Geometry check sheet. Reference: the model listing, model coordinates, mm. A direction names the side the tool comes from. Coordinates: 2 decimals unless noted, no trailing zeros. Write each loop counter-clockwise with the first axis right and the second up, starting at its lowest first coordinate (ties: lowest second). Pieces come first, ordered by that corner, then holes. Notation, with made-up numbers: (12.5, 36) -> (31.5, 36) arc R13 cw to (31.5, 48) -> close; hole circle Ø1 at (73, -22). An arc over 180 degrees is marked (long way). One line per question, with ' | ' between items.
```python
from build123d import *

# Parameters (mm, degrees)
F0_W     = 50.8
F0_H     = 50.8
F1_DEPTH = 50.8
F2_W     = 25.4
F2_H     = 25.4
F3_DEPTH = 12.7
F4_R     = 11
F5_DEPTH = 50.8
F6_R     = 11
F7_DEPTH = 12.7


with BuildPart() as f1:
    # F0 (on Front) → F1 (new body)
    with BuildSketch(Plane.XZ):
        with Locations((-21.93247, 21.290337)):
            Rectangle(F0_W, F0_H)
    extrude(amount=F1_DEPTH)

    # F2 (on face) → F3 (join)
    with BuildSketch(Plane.XZ.offset(50.8)):
        with Locations((-20.790899, 21.946741)):
            Rectangle(F2_W, F2_H)
    extrude(amount=F3_DEPTH)

    # F4 (on face) → F5 (cut)
    with BuildSketch(Plane.XY.offset(46.690337)):
        with Locations((-23.502136, -23.116853)):
            Circle(F4_R)
    extrude(amount=-F5_DEPTH, mode=Mode.SUBTRACT)

    # F6 (on face) → F7 (join)
    with BuildSketch(Plane(origin=(-47.33247, 0, 0), x_dir=(0, -1, 0), z_dir=(-1, 0, 0))):
        with Locations((24.015844, 23.116853)):
            Circle(F6_R)
    extrude(amount=F7_DEPTH)


solid = f1.part
```
(1) Tool access check on faces 4 (the face through (-8.091, -57, 22)), 5 (the face through (-33.491, -57, 22)), 6 (the face through (-53.594, -34.177, 18.904)). Record the directions out of +Z, -Z, +X, -X, +Y, -Y that give a thin tool (end or side, any length) a straight path to the whole face; none if there is none.
Answers below:
face 4: +Z, -Z, +X, -Y | face 5: +Z, -Z, -X, -Y | face 6: -X
(2) Cross-section at A-A (y = -27). Record the cut outline in (x, z), plus the area to 3 significant figures.
Answers below:
outline: (-60.03, 12.53) -> (-47.33, 12.53) -> (-47.33, -4.11) -> (-33.79, -4.11) -> (-33.79, 46.69) -> (-47.33, 46.69) -> (-47.33, 33.7) -> (-60.03, 33.7) -> close; (-13.21, -4.11) -> (3.47, -4.11) -> (3.47, 46.69) -> (-13.21, 46.69) -> close | area: 1,800 mm²
(3) Draft check along X on faces 1 (the face through (-25.887, -33.855, 21.646)), 2 (the face through (-21, -57, 34.647)), 3 (the face through (-60.032, -24, 23)). Enter one of: pulls with the +X half, pulls with the -X half, needs draft (parallel to the pull), parting line crosses it, or undercut.
Answers below:
face 1: undercut | face 2: needs draft | face 3: pulls with the -X half
(4) Depth check by flat-ended pin: P1, Ø2, axis at y = -37.5, z = 9, coming from the -X side; P2, Ø4, axis at x = -7.5, z = 3, coming from the -Y side; P3, Ø4, axis at y = -60, z = 25.5, coming from the -X side. Enter the tip coordinate at first touch or a pass-through.
Answers below:
P1: stops at x = -47.33 | P2: stops at y = -50.8 | P3: stops at x = -33.49
(5) Cross-section at D-D (x = -38.5). Record the cut outline in (y, z).
Answers below:
outline: (-50.8, -4.11) -> (0, -4.11) -> (0, 46.69) -> (-50.8, 46.69) -> close
(6) Cross-section at B-B (x = -26). Record the cut outline in (y, z), plus the area to 3 significant figures.
Answers below:
outline: (-63.5, 9.25) -> (-50.8, 9.25) -> (-50.8, -4.11) -> (-33.83, -4.11) -> (-33.83, 46.69) -> (-50.8, 46.69) -> (-50.8, 34.65) -> (-63.5, 34.65) -> close; (-12.4, -4.11) -> (0, -4.11) -> (0, 46.69) -> (-12.4, 46.69) -> close | area: 1,810 mm²
(7) Material ranges on line 1 (Y direction, x = -23, z = 27); line 2 (X direction, y = -8, z = 9); line 3 (Y direction, x = -15.5, z = 32.5), recorded low to high.
Answers below:
line 1: y = -63.5 to -34.11, -12.13 to 0 | line 2: x = -47.33 to 3.47 | line 3: y = -63.5 to -30.66, -15.57 to 0
(8) Cross-section at C-C (z = 28). Record the cut outline in (x, y), plus the area to 3 significant figures.
Answers below:
outline: (-60.03, -33.87) -> (-47.33, -33.87) -> (-47.33, -50.8) -> (-33.49, -50.8) -> (-33.49, -63.5) -> (-8.09, -63.5) -> (-8.09, -50.8) -> (3.47, -50.8) -> (3.47, 0) -> (-47.33, 0) -> (-47.33, -14.16) -> (-60.03, -14.16) -> close; hole circle Ø22 at (-23.5, -23.12) | area: 2,770 mm²
